from build123d import *

# Parameters (mm, degrees)
SKETCH1_W           = 30
SKETCH1_H           = 30
BOSS_EXTRUDE1_DEPTH = 5
SKETCH2_R           = 3.175
CUT_EXTRUDE1_DEPTH  = 5
SKETCH3_RX          = 2.25
SKETCH3_RY          = 1.75
CUT_EXTRUDE3_DEPTH  = 30


with BuildPart() as part:
    # Sketch1 → Boss-Extrude1 (new body)
    with BuildSketch(Plane(origin=(0, 0, 0), x_dir=(1, 0, 0), z_dir=(0, 1, 0))):
        with Locations((-15, -15)):
            Rectangle(SKETCH1_W, SKETCH1_H)
    extrude(amount=BOSS_EXTRUDE1_DEPTH)

    # Sketch2 → Cut-Extrude1 (cut)
    with BuildSketch(Plane(origin=(0, 5, 0), x_dir=(1, 0, 0), z_dir=(0, 1, 0))):
        with Locations((-15, -15)):
            Circle(SKETCH2_R)
    extrude(amount=-CUT_EXTRUDE1_DEPTH, mode=Mode.SUBTRACT)

    # Sketch3 → Cut-Extrude3 (cut)
    with BuildSketch(Plane.XY.offset(30)):
        with Locations(Location((-24.0875, 5), (0, 0, 180))):
            Ellipse(SKETCH3_RX, SKETCH3_RY)
        with Locations(Location((-5.9125, 5), (0, 0, 180))):
            Ellipse(SKETCH3_RX, SKETCH3_RY)
    extrude(amount=-CUT_EXTRUDE3_DEPTH, mode=Mode.SUBTRACT)


solid = part.part
Part model, mm, in its own coordinate system. Give positions to 0.01 mm unless a question says otherwise; leave off trailing zeros. Order: outer loops, then holes, each group sorted by start corner. A loop starts at its lowest first (then second) coordinate and runs counter-clockwise, first axis right, second up. Notation, with made-up numbers: (19, -22.5) - (34, -22.5) arc R22 cw to (34, -2.5) - close; hole circle Ø7 at (62.5, -31). An arc over 180 degrees is marked (long way). Use a Markdown table: item, result.
1) Saw through at A-A on x = -15. List the corners of the cut face in (y, z) (3 decimals), plus the area to 3 significant figures.
Checked values:
| item | result |
|---|---|
| outline | (0, 0) - (5, 0) - (5, 11.825) - (0, 11.825) - close; (0, 18.175) - (5, 18.175) - (5, 30) - (0, 30) - close |
| area | 118 mm² |
2) Saw through at B-B on y = 1.05. List the corners of the cut face in (x, z) (3 decimals).
Checked values:
| item | result |
|---|---|
| outline | (-30, 0) - (0, 0) - (0, 30) - (-30, 30) - close; hole circle Ø6.35 at (-15, 15) |
3) Two-plate mould, pull along X, no slides. Class faces 1 (the flat face through (0, 2, 15)), 2 (the cylindrical face through (-11.97, 2.54, 14.05)), 3 (the flat face through (-2, 5, 15)), 4 (the flat face through (-30, 2, 15)): +X half, -X half, draft (parallel to the pull), parting line (faces both ways), or undercut.
Checked values:
| item | result |
|---|---|
| face 1 | +X half |
| face 2 | undercut |
| face 3 | draft |
| face 4 | -X half |
4) Probe L1, parallel to Z at x = -15, y = 3.35 (3 decimals); L2, parallel to X at y = 3.9, z = 15 (3 decimals); L3, parallel to X at y = 4.5, z = 26.5. List the from-to ranges inside material, lowest first. Write a range as from..to.
Checked values:
| item | result |
|---|---|
| L1 | 0..11.825, 18.175..30 |
| L2 | -30..-25.837, -22.338..-18.175, -11.825..-7.662, -4.163..0 |
| L3 | -30..-26.24, -21.93..-8.07, -3.76..0 |
